from build123d import *

# Parameters (mm, degrees)
F1_DEPTH = 50
F3_DEPTH = 50
F4_R     = 1.5
F5_DEPTH = 15.001


with BuildPart() as f1:
    # F0 (on Top) → F1 (new body)
    with BuildSketch(Plane.XY):
        with BuildLine():
            ThreePointArc((-25, -5.664544), (0, 0), (25, -5.664544))
            Line((25, -5.664544), (25, 9.335456))
            Line((25, 9.335456), (-25, 9.335456))
            Line((-25, 9.335456), (-25, -5.664544))
        make_face()
    extrude(amount=F1_DEPTH)

    # F2 (on face) → F3 (join, through all)
    with BuildSketch(Plane.YZ.offset(25)):
        with BuildLine():
            ThreePointArc((9.335456, 50), (16.835456, 57.5), (24.335456, 50))
            Line((24.335456, 50), (24.335456, 35))
            Line((24.335456, 35), (29.335456, 35))
            Line((29.335456, 35), (29.335456, 50))
            ThreePointArc((29.335456, 50), (16.835456, 62.5), (4.335456, 50))
            Line((4.335456, 50), (9.335456, 50))
        make_face()
    extrude(amount=-F3_DEPTH)

    # F4 (on face) → F5 (cut, through all)
    with BuildSketch(Plane(origin=(0, 9.335456, 0), x_dir=(-1, 0, 0), z_dir=(0, 1, 0))):
        with Locations((-16, 21.5)):
            Circle(F4_R)
        with Locations((0, 21.5)):
            Circle(F4_R)
        with Locations((16, 21.5)):
            Circle(F4_R)
        with Locations((16, 5.5)):
            Circle(F4_R)
        with Locations((0, 5.5)):
            Circle(F4_R)
        with Locations((-16, 5.5)):
            Circle(F4_R)
    extrude(amount=-F5_DEPTH, mode=Mode.SUBTRACT)


solid = f1.part
Geometry: final body of the model. Coordinates: model frame, mm. A direction names the side the tool comes from. Coordinates: 2 decimals unless noted, no trailing zeros. Order: outer loops, then holes, each group sorted by start corner. A loop starts at its lowest first (then second) coordinate and runs counter-clockwise, first axis right, second up.
1) Section B-B (z = 54.5). Return loops of the section in (x, y).
Result sheet:
outline: (-25, 5.17) - (25, 5.17) - (25, 10.84) - (-25, 10.84) - close; (-25, 22.84) - (25, 22.84) - (25, 28.5) - (-25, 28.5) - close
2) Set-up query: faces 5 (the flat face through (25, 8, 32)), 6 (the cylindrical face through (-17.43, 3.4, 21.95)), 7 (the flat face through (0, 2, 50)), 8 (the flat face through (0, 27, 35)), 9 (the flat face through (0, 24.335, 43)). Return all of +Z, -Z, +X, -X, +Y, -Y with unobstructed straight access to the full face (end or side cutting, diameter ignored); none if empty.
Result sheet:
face 5: +Z, -Z, +X, +Y, -Y
face 6: +Y, -Y
face 7: +Z, +X, -X, -Y
face 8: -Z, +X, -X, +Y
face 9: -Z, +X, -X
3) Draft query along Y for faces 1 (the flat face through (0, 29.335, 42)), 2 (the cylindrical face through (0, 0, 25)), 3 (the flat face through (0, 4, 0)), 4 (the flat face through (0, 9.335, 25)). Return one class per face: released by +Y, released by -Y, zero draft, split by the parting line, or undercut.
Result sheet:
face 1: released by +Y
face 2: released by -Y
face 3: zero draft
face 4: undercut
4) Section A-A (x = 0). Return loops of the section in (y, z), then the cut area to 3 significant figures.
Result sheet:
outline: (0, 0) - (9.34, 0) - (9.34, 4) - (0, 4) - close; (0, 7) - (9.34, 7) - (9.34, 20) - (0, 20) - close; (0, 23) - (9.34, 23) - (9.34, 50) arc R7.5 cw to (24.34, 50) - (24.34, 35) - (29.34, 35) - (29.34, 50) arc R12.5 ccw to (4.34, 50) - (0, 50) - close
area: 643 mm2
5) Section D-D (x = 20.5). Return loops of the section in (y, z), then the cut area to 3 significant figures.
Result sheet:
outline: (-3.74, 0) - (9.34, 0) - (9.34, 50) arc R7.5 cw to (24.34, 50) - (24.34, 35) - (29.34, 35) - (29.34, 50) arc R12.5 ccw to (4.34, 50) - (-3.74, 50) - close
area: 886 mm2
6) Section C-C (z = 5.5). Return loops of the section in (x, y), then the cut area to 3 significant figures.
Result sheet:
outline: (-25, -5.66) arc R58 cw to (-17.5, -2.7) - (-17.5, 9.34) - (-25, 9.34) - close; (-14.5, -1.84) arc R58 cw to (-1.5, -0.02) - (-1.5, 9.34) - (-14.5, 9.34) - close; (1.5, -0.02) arc R58 cw to (14.5, -1.84) - (14.5, 9.34) - (1.5, 9.34) - close; (17.5, -2.7) arc R58 cw to (25, -5.66) - (25, 9.34) - (17.5, 9.34) - close
area: 462 mm2
7) Ray query, probe 1 along X at (y, z) = (5, 21.5); probe 2 along Z at (x, y) = (-16, 0); probe 3 along Y at (x, z) = (-1.5, 42). Return the intervals inside material, ascending.
Result sheet:
probe 1: x = -25 to -17.5, -14.5 to -1.5, 1.5 to 14.5, 17.5 to 25
probe 2: z = 0 to 4, 7 to 20, 23 to 50
probe 3: y = -0.02 to 9.34, 24.34 to 29.34
8) First-contact query: P1, Ø4, axis at x = 1.5, y = 25.5, coming from the -Z side; P2, Ø16.5, axis at x = -5, z = 41, coming from the -Y side; P3, Ø4, axis at x = -16, z = 21.5, coming from the +Y side. Flat tips, straight axial feed; report the tip coordinate or a pass-through.
Result sheet:
P1: stops at z = 35
P2: stops at y = -1.53
P3: stops at y = 9.34
